CAD build for the part. Positions are in the model's coordinates, mm. Face numbers are marked on the shaded views. A direction names the side the tool comes from. Round coordinates to 2 decimals unless told otherwise and drop trailing zeros. Order: outer loops, then holes, each group sorted by start corner. A loop starts at its lowest first (then second) coordinate and runs counter-clockwise, first axis right, second up. Notation, with made-up numbers: (33.5, 22) -> (56.5, 22) arc R25 cw to (56.5, 44) -> close; hole circle Ø1 at (0, 17). An arc over 180 degrees is marked (long way). Return JSON: item names as keys, results as strings. Group by question number.
Q1. Mould opens along Z. For the marked faces 1, 2 and 3 say: +Z half, -Z half, draft (parallel to the pull), parting line (faces both ways), or undercut.
Q2. Flat gauge pins, fed straight in: pin 1 (1 mm diameter, centred on x = 2.5, z = -6, fed in from +Y); pin 2 (2.5 mm diameter, centred on x = 1.5, z = 4, fed in from -Y); pin 3 (5 mm diameter, centred on x = -3, y = -0.5, fed in from -Z); pin 4 (1 mm diameter, centred on x = 3, y = 4, fed in from +Z). Where does each tip first touch, or does it go through?
Q3. Cut at A-A (z = -2.25). Write the cut outline in (x, y).
Q4. Probe line 1 along Y through (x, z) = (0, -3.5); line 2 along Y through (x, z) = (2.75, 2.5); line 3 along Z through (x, y) = (-2, -0.5). List the from-to ranges inside material, lowest first.
Q5. Which spindle directions (+Z, -Z, +X, -X, +Y, -Y) get a long thin tool onto all of the face, cutting with end or side? Do the marked faces 4 and 5. Say none if no direction does.
Autodesk Inventor part; units mm, degrees
ref_plane "WorkPlane11" through (0, 0, 0) normal (0, 0, 1) x (1, 0, 0)
ref_plane "Work Plane2" through (0, 0, -5.7) normal (0, 0, 1) x (1, 0, 0)
ref_plane "WorkPlane9" through (0, 0, 8.3) normal (0, 0, 1) x (1, 0, 0)
ref_plane "WorkPlane11" through (0, 0, 0) normal (0, 0, 1) x (1, 0, 0)
ref_plane "Work Plane2" through (0, 0, -5.7) normal (0, 0, 1) x (1, 0, 0)
ref_plane "WorkPlane9" through (0, 0, 8.3) normal (0, 0, 1) x (1, 0, 0)
sketch "Sketch1" plane through (0, 0, 0) normal (0, 0, 1) x (1, 0, 0)
  point P0 (0, 0)
sketch "Sketch2" plane through (0, 0, 0) normal (0, 0, 1) x (1, 0, 0)
  circle A0 centre (0, 0) radius 2.75
  dimension "d2" = 5.5
extrude "Extrusion1" add sketch "Sketch2" against normal blind 0.75
sketch "Sketch3" plane through (0, 0, -0.75) normal (0, 0, -1) x (-1, 0, 0)
  circle A0 centre (0, 0) radius 3
  circle A1 centre (0, 0) radius 2.75 construction
  dimension "d8" = 6
extrude "Extrusion2" add sketch "Sketch3" along normal blind 7.95
sketch "Sketch4" plane through (0, 0, 0) normal (0, 0, 1) x (1, 0, 0)
  circle A0 centre (0, 0) radius 5.65
  circle A1 centre (0, 0) radius 2.75 construction
  dimension "d12" = 11.3
extrude "Extrusion3" add sketch "Sketch4" along normal blind 3.3
sketch "Sketch5" plane through (0, 0, 0) normal (0, 1, 0) x (-1, 0, 0)
  line L0 (5.65, 0) -> (2.75, 0)
  line L1 (5.65, 2.9) -> (5.65, 0)
  line L2 (2.75, 0) -> (5.65, 2.9)
  line L3 (-5.65, 0) -> (5.65, 0) construction
  line L4 (0, -7.649262) -> (0, 5.899262)
  line L5 (0, -10.358967) -> (0, 8.608967)
  line L6 (5.65, 0) -> (5.65, 3.3)
  line L7 (-4.75, 0) -> (4.75, 0)
  line L8 (2.75, 0) -> (2.75, -0.75)
  dimension "d17" = 45
revolve "Revolution1" cut sketch "Sketch5" angle 360 about axis through (0, 0, -7.649262) along (0, 0, 1)
sketch "Sketch6" plane through (0, 0, 0) normal (0, 1, 0) x (-1, 0, 0)
  line L0 (0, 3.3) -> (0, 4.713334)
  line L1 (0, 3.3) -> (5.65, 3.3)
  arc A0 (5.65, 3.3) -> (0, 4.713334) centre (0, -7.286666) ccw
  line L2 (-5.65, 3.3) -> (5.65, 3.3) construction
  line L3 (0, -7.649262) -> (0, 5.899262)
  line L4 (0, -10.358967) -> (0, 8.608967)
  line L5 (5.65, 2.9) -> (5.65, 3.3)
  arc A1 (0, 4.713334) -> (-5.65, 3.3) centre (0, -7.286666) ccw
  dimension "d20" = 12
  dimension "d24" = 5.65
revolve "Revolution2" add sketch "Sketch6" angle 360 about axis through (0, 0, -7.649262) along (0, 0, 1)
fillet "Fillet1" radius 1.5 2 edges at (0, 2.75, 0) (0, -2.75, 0)
chamfer "Chamfer1" distance 1.25 distance2 0.25 1 edges at (3, 0, -0.75) measured on face at (-2.9612, -0.4812, -6.05)
sketch "Sketch8" plane through (0, 0, 0) normal (0, 1, 0) x (-1, 0, 0)
  line L0 (-5.65, 4.713334) -> (5.65, 4.713334)
  line L1 (5.65, 4.713334) -> (5.65, 2.313334)
  line L2 (5.65, 2.313334) -> (-5.65, 2.313334)
  line L3 (-5.65, 2.313334) -> (-5.65, 4.713334)
  arc A0 (5.65, 3.3) -> (-5.65, 3.3) centre (0, -7.286666) ccw
  line L4 (-5.65, 2.9) -> (-5.65, 3.3)
  line L5 (5.65, 2.9) -> (5.65, 3.3)
  dimension "msp_d31" = 2.4
extrude "Extrusion4" cut sketch "Sketch8" against normal mid plane 1.6
thread "Thread1"
ref_plane "MSC_PF1" through (0, 0, 0) normal (1, 0, 0) x (0, 1, 0)
ref_plane "MSC_PT1" through (-5.65, 0, 2.9) normal (0, 0, -1) x (-1, 0, 0)
equation "\"d28\" = r"
equation "\"d29\" = msp_x"
equation "\"d30\" = 0.25 * PTC"
equation "\"d3\" = -msp_x + ParA"
equation "\"d8\" = NND"
equation "\"d9\" = msp_x - ParK + NLG - ParA"
equation "\"d12\" = Dk"
equation "\"d13\" = ParK"
equation "\"msp_d31\" = ParT"
equation "\"msp_d32\" = ParN"
equation "\"d2\" = 0.5 * PTC + msp_mdtds"
equation "\"d20\" = rf"
equation "\"d24\" = 0.5 * Dk"
equation "\"PTC\" = 1"
equation "\"NND\" = 6"
equation "\"msp_x\" = 1.25 * PTC"
equation "\"NLG\" = 12"
equation "\"msp_mdtds\" = NND - PTC"
equation "\"ParK\" = 3.3"
equation "\"ParN\" = 1.6"
equation "\"ParT\" = 2.4"
equation "\"r\" = 1.5"
equation "\"prf_c\" = 0"
equation "\"ParA\" = 2"
equation "\"Dk\" = 11.3"
equation "\"rf\" = 12"
equation "\"ParF\" = 1.4"
equation "\"THREADDIA\" = NND"
equation "\"PG\" = 1.2345"
equation "\"TEMPLATE\" = 1.2345"
properties part number "ISO 2010 - M6x12" material "Stainless Steel, 440C"
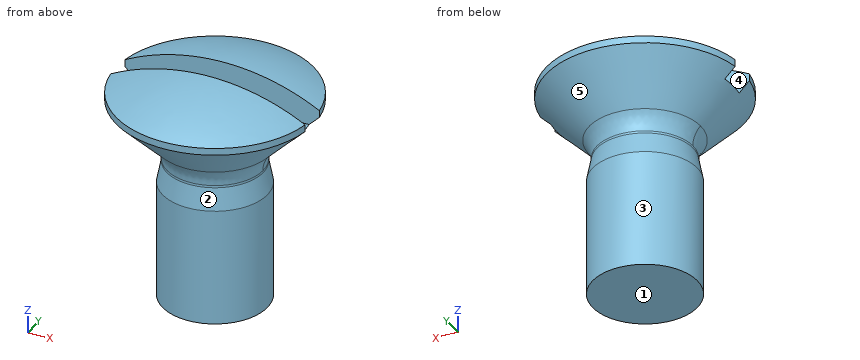
Solution:
{
 "1": {"face 1": "-Z half", "face 2": "undercut", "face 3": "draft"},
 "2": {"pin 1": "stops at y = 2.24", "pin 2": "stops at y = -5.63", "pin 3": "stops at z = -8.7", "pin 4": "stops at z = 3.84"},
 "3": {"outline": "circle Ø6 at (0, 0)"},
 "4": {"line 1": "y = -3 to 3", "line 2": "y = -4.47 to -0.8, 0.8 to 4.47", "line 3": "z = -8.7 to 2.31"},
 "5": {"face 4": "+Z, +X, -X", "face 5": "-Z"}
}
